The drawing under review shows one solid part. Ordinate dimensions are in mm from its lowest x, y, z. A direction names the side the tool comes from. Coordinates: 2 decimals unless noted, no trailing zeros. Order: outer loops, then holes, each group sorted by start corner. A loop starts at its lowest first (then second) coordinate and runs counter-clockwise, first axis right, second up.
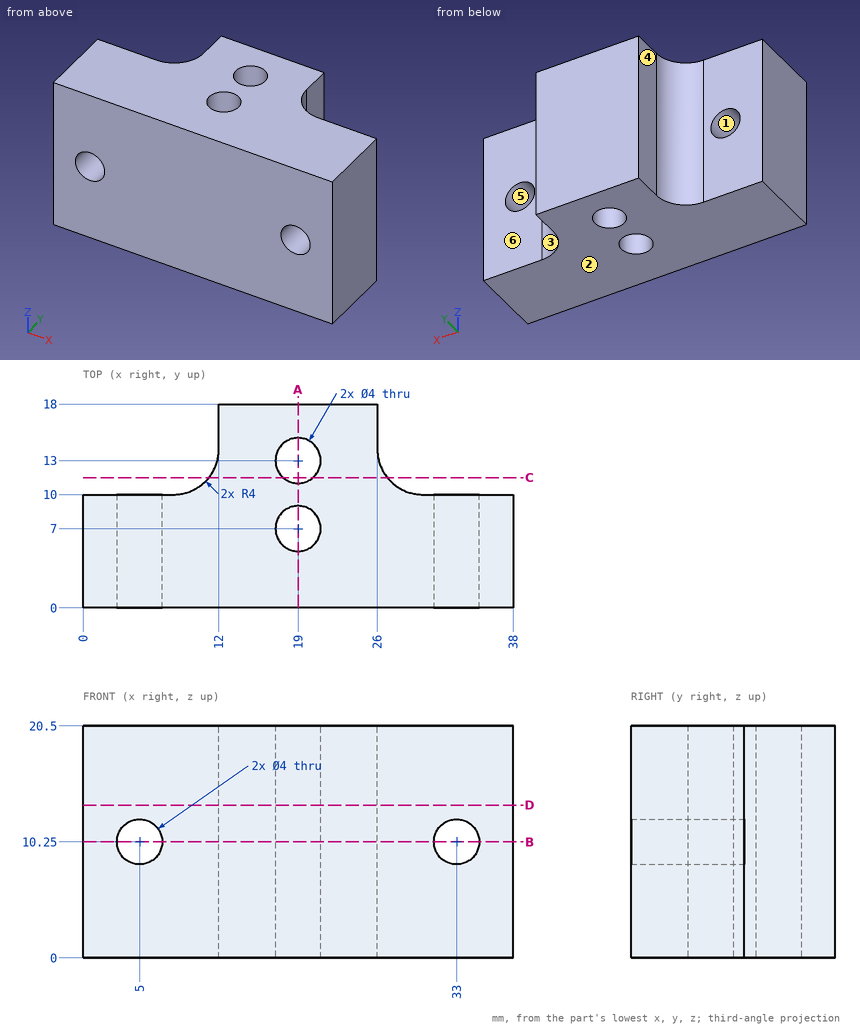
1. For the marked faces 4, 5 and 6, list the 3-axis set-ups (+Z, -Z, +X, -X, +Y, -Y) from which the entire face can be reached by the end or side of a thin tool; tool diameter is ignored.
2. Add section A-A (x = 19). Give the boundary of the cut face in (y, z), and give its area (3 significant figures).
3. Add section C-C (y = 11.5). Give the boundary of the cut face in (x, z).
4. Mouldability with a two-part tool opening along Z and no side actions: class the marked faces 1, 2 and 3 as pulls with the +Z half, pulls with the -Z half, needs draft (parallel to the pull), parting line crosses it, or undercut.
5. Add section D-D (z = 13.5). Give the boundary of the cut face in (x, y).
6. Add section B-B (z = 10.25). Give the boundary of the cut face in (x, y).
7. Insertion check: pin 1 (4.5 mm diameter, centred on y = 17, z = 6.5, fed in from -X); pin 2 (3 mm diameter, centred on x = 14.5, z = 9, fed in from -Y); pin 3 (1.2 mm diameter, centred on y = 16, z = 8, fed in from +X); pin 4 (2 mm diameter, centred on y = 13.5, z = 6, fed in from +X). Each pin has a flat end and moves straight along its axis. Give the tip position at first contact, or say it passes through.
8. To check wall thickness, follow line 1 (Y direction, x = 19, z = 7); line 2 (Z direction, x = 5, y = 5.75); line 3 (Y direction, x = 32, z = 1.5). State the ranges of each line that lie inside material, in increasing order.
Solution:
1. face 4: +Z, -Z, -X, +Y
1. face 5: +Y, -Y
1. face 6: +Z, -Z, +X, +Y
2. outline: (0, 0) - (5, 0) - (5, 20.5) - (0, 20.5) - close; (9, 0) - (11, 0) - (11, 20.5) - (9, 20.5) - close; (15, 0) - (18, 0) - (18, 20.5) - (15, 20.5) - close
2. area: 205 mm2
3. outline: (11.12, 0) - (17.68, 0) - (17.68, 20.5) - (11.12, 20.5) - close; (20.32, 0) - (26.88, 0) - (26.88, 20.5) - (20.32, 20.5) - close
4. face 1: undercut
4. face 2: pulls with the -Z half
4. face 3: needs draft
5. outline: (0, 0) - (38, 0) - (38, 10) - (30, 10) arc R4 cw to (26, 14) - (26, 18) - (12, 18) - (12, 14) arc R4 cw to (8, 10) - (0, 10) - close; hole circle Ø4 at (19, 7); hole circle Ø4 at (19, 13)
6. outline: (0, 0) - (3, 0) - (3, 10) - (0, 10) - close; (7, 0) - (31, 0) - (31, 10) - (30, 10) arc R4 cw to (26, 14) - (26, 18) - (12, 18) - (12, 14) arc R4 cw to (8, 10) - (7, 10) - close; (35, 0) - (38, 0) - (38, 10) - (35, 10) - close; hole circle Ø4 at (19, 7); hole circle Ø4 at (19, 13)
7. pin 1: stops at x = 12
7. pin 2: stops at y = 0
7. pin 3: stops at x = 26
7. pin 4: stops at x = 26.29
8. line 1: y = 0 to 5, 9 to 11, 15 to 18
8. line 2: z = 0 to 8.25, 12.25 to 20.5
8. line 3: y = 0 to 10
